Geometry check sheet. Reference: the model listing, model coordinates, mm. Give positions to 0.01 mm unless a question says otherwise; leave off trailing zeros. Write each loop counter-clockwise with the first axis right and the second up, starting at its lowest first coordinate (ties: lowest second). Pieces come first, ordered by that corner, then holes. Notation, with made-up numbers: M -4.75,54 L 24.25,54 A12 cw 24.25,61 Z; hole C 24,87 d4. An arc over 180 degrees is marked long. One line per item, written item: value. Start each with the question number.
1. Release check for a two-part mould opening along Z. For faces 1 (the face through (237.972, 4.93, -11.406)), 2 (the face through (138.82, 4.93, -80.81)), 3 (the face through (106, 5, -150)), 4 (the face through (250, 5, -75)) record: pulls with the +Z half, pulls with the -Z half, needs draft (parallel to the pull), parting line crosses it, or undercut.
2. Gauge pin test, flat ends, axial feed: pin 1 (2 mm diameter, centred on y = 6.5, z = -27, fed in from +X); pin 2 (10 mm diameter, centred on x = 219, z = -109, fed in from -Y); pin 3 (3 mm diameter, centred on x = 50, z = -144.82, fed in from -Y); pin 4 (6 mm diameter, centred on y = 3, z = -134, fed in from +X). Record the tip position at first contact, or that the pin passes through.
3. Cross-section at A-A on x = 150. Record the cut outline in (y, z).
4. Cross-section at B-B on y = 4.75. Count the separate pieces of the cut face and the enclosed holes in it, then the cut area to 3 significant figures.
5. Scan lines: line 1 (X direction, y = 4, z = -109.82); line 2 (Z direction, x = 242.34, y = 2.75); line 3 (X direction, y = 6, z = -75). Record each from-to range of solid material in increasing order.
from build123d import *

# Parameters (mm, degrees)
BOSS_EXTRUDE1_DEPTH = 10
SKETCH2_R           = 12.59794853
CUT_EXTRUDE1_DEPTH  = 292.719042916
SKETCH3_R           = 2
CUT_EXTRUDE10_DEPTH = 292.719042916
SKETCH4_R           = 2
CUT_EXTRUDE11_DEPTH = 292.719042916
SKETCH5_R           = 2
CUT_EXTRUDE12_DEPTH = 292.719042916
SKETCH6_R           = 2
CUT_EXTRUDE13_DEPTH = 292.719042916
SKETCH10_R          = 2
CUT_EXTRUDE15_DEPTH = 292.719042916
SKETCH11_R          = 2
CUT_EXTRUDE16_DEPTH = 292.719042916


with BuildPart() as part:
    # Sketch1 → Boss-Extrude1 (new body)
    with BuildSketch(Plane(origin=(0, 0, 0), x_dir=(1, 0, 0), z_dir=(0, 1, 0))):
        with BuildLine():
            Line((0, 0), (210, 0))
            ThreePointArc((210, 0), (238.284271247, 11.715728753), (250, 40))
            Line((250, 40), (250, 110))
            ThreePointArc((250, 110), (238.284271247, 138.284271247), (210, 150))
            Line((210, 150), (0, 150))
            Line((0, 150), (0, 0))
        make_face()
    extrude(amount=BOSS_EXTRUDE1_DEPTH)

    # Sketch2 → Cut-Extrude1 (cut, through all)
    with BuildSketch(Plane.XZ):
        with Locations(Location((150, -75, 0), (0, 0, 270))):
            Circle(SKETCH2_R)
    extrude(amount=-CUT_EXTRUDE1_DEPTH, mode=Mode.SUBTRACT)

    # Sketch3 → Cut-Extrude10 (cut, through all)
    with BuildSketch(Plane(origin=(0, 10, 0), x_dir=(1, 0, 0), z_dir=(0, 1, 0))):
        with Locations(Location((6.310878228, 144.817130454, 0), (0, 0, 270))):
            Circle(SKETCH3_R)
    extrude(amount=-CUT_EXTRUDE10_DEPTH, mode=Mode.SUBTRACT)

    # Sketch4 → Cut-Extrude11 (cut, through all)
    with BuildSketch(Plane(origin=(0, 10, 0), x_dir=(1, 0, 0), z_dir=(0, 1, 0))):
        with Locations(Location((5.635720357, 4.632829204, 0), (0, 0, 270))):
            Circle(SKETCH4_R)
    extrude(amount=-CUT_EXTRUDE11_DEPTH, mode=Mode.SUBTRACT)

    # Sketch5 → Cut-Extrude12 (cut, through all)
    with BuildSketch(Plane(origin=(0, 10, 0), x_dir=(1, 0, 0), z_dir=(0, 1, 0))):
        with Locations(Location((226.364130141, 140.421237055, 0), (0, 0, 270))):
            Circle(SKETCH5_R)
    extrude(amount=-CUT_EXTRUDE12_DEPTH, mode=Mode.SUBTRACT)

    # Sketch6 → Cut-Extrude13 (cut, through all)
    with BuildSketch(Plane(origin=(0, 10, 0), x_dir=(1, 0, 0), z_dir=(0, 1, 0))):
        with Locations(Location((228.949949788, 12.164582591, 0), (0, 0, 270))):
            Circle(SKETCH6_R)
    extrude(amount=-CUT_EXTRUDE13_DEPTH, mode=Mode.SUBTRACT)

    # Sketch10 → Cut-Extrude15 (cut, through all)
    with BuildSketch(Plane(origin=(0, 10, 0), x_dir=(1, 0, 0), z_dir=(0, 1, 0))):
        with Locations(Location((50, 144.82, 0), (0, 0, 270))):
            Circle(SKETCH10_R)
        with Locations(Location((50, 4.63, 0), (0, 0, 270))):
            Circle(SKETCH10_R)
        with Locations(Location((100, 4.63, 0), (0, 0, 270))):
            Circle(SKETCH10_R)
        with Locations(Location((100, 144.82, 0), (0, 0, 270))):
            Circle(SKETCH10_R)
        with Locations(Location((50, 109.82, 0), (0, 0, 270))):
            Circle(SKETCH10_R)
        with Locations(Location((50, 54.63, 0), (0, 0, 270))):
            Circle(SKETCH10_R)
    extrude(amount=-CUT_EXTRUDE15_DEPTH, mode=Mode.SUBTRACT)

    # Sketch11 → Cut-Extrude16 (cut, through all)
    with BuildSketch(Plane(origin=(0, 10, 0), x_dir=(1, 0, 0), z_dir=(0, 1, 0))):
        with Locations(Location((242.34, 83, 0), (0, 0, 270))):
            Circle(SKETCH11_R)
        with Locations(Location((242.34, 67, 0), (0, 0, 270))):
            Circle(SKETCH11_R)
    extrude(amount=-CUT_EXTRUDE16_DEPTH, mode=Mode.SUBTRACT)


solid = part.part
Report:
1. face 1: pulls with the +Z half
1. face 2: undercut
1. face 3: pulls with the -Z half
1. face 4: needs draft
2. pin 1: stops at x = 248.16
2. pin 2: stops at y = 0
2. pin 3: passes through
2. pin 4: stops at x = 244.04
3. outline: M 0,-150 L 10,-150 L 10,-87.6 L 0,-87.6 Z; M 0,-62.4 L 10,-62.4 L 10,0 L 0,0 Z
4. separate pieces: 1
4. enclosed holes: 13
4. area: 36,200 mm^2
5. line 1: x = 0 to 48, 52 to 250
5. line 2: z = -133.54 to -85, -81 to -69, -65 to -16.46
5. line 3: x = 0 to 137.4, 162.6 to 250
